Geometry check sheet. Reference: the model listing, model coordinates, mm. Face numbers are marked on the shaded views. A direction names the side the tool comes from. Give positions to 0.01 mm unless a question says otherwise; leave off trailing zeros. Write each loop counter-clockwise with the first axis right and the second up, starting at its lowest first coordinate (ties: lowest second). Pieces come first, ordered by that corner, then holes. Notation, with made-up numbers: M 28.5,51.25 L 34.5,51.25 A25 cw 34.5,66.25 Z; hole C 62,50.5 d7. An arc over 180 degrees is marked long. One line per item, written item: value. Start each with the question number.
1. Tool access check on the marked faces 4, 5 and 6. Record the directions out of +Z, -Z, +X, -X, +Y, -Y that give a thin tool (end or side, any length) a straight path to the whole face; none if there is none.
2. Cross-section at A-A on y = -9. Count the separate pieces of the cut face and the enclosed holes in it, then the cut area to 3 significant figures.
3. Cross-section at C-C on z = 7.5. Record the cut outline in (x, y).
4. Gauge pin test, flat ends, axial feed: pin 1 (4 mm diameter, centred on x = 22, y = -3.5, fed in from -Z); pin 2 (1.5 mm diameter, centred on x = -16.5, y = -9, fed in from +Z); pin 3 (1.5 mm diameter, centred on x = -6.5, y = -10, fed in from -Z). Record the tip position at first contact, or that the pin passes through.
5. Cross-section at B-B on x = 4.5. Record the cut outline in (y, z).
6. Scan lines: line 1 (X direction, y = -6.35, z = -7.3); line 2 (X direction, y = -6.35, z = -7.4); line 3 (X direction, y = -7.25, z = -8). Record each from-to range of solid material in increasing order.
7. Cross-section at D-D on z = 11.25. Record the cut outline in (x, y).
8. Release check for a two-part mould opening along X. For the marked faces 1, 2 and 3 record: pulls with the +X half, pulls with the -X half, needs draft (parallel to the pull), parting line crosses it, or undercut.
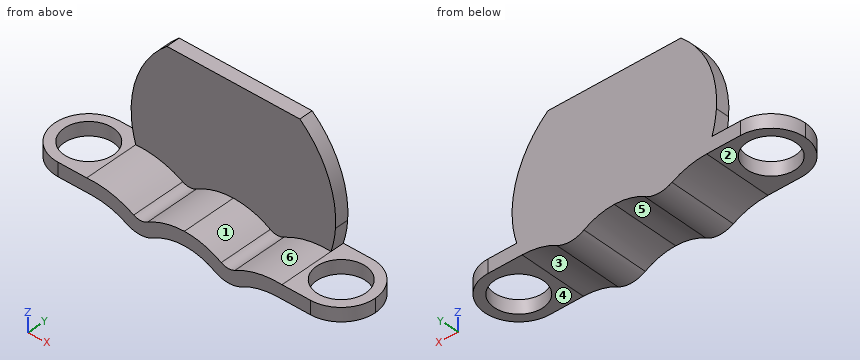
from build123d import *

# Parameters (mm, degrees)
F1_DEPTH = 2.54
F2_DEPTH = 12.7
F3_R     = 5.08
F5_DEPTH = 25.4
F7_R     = 2.54


with BuildPart() as f1:
    # F0 (on Front) → F1 (new body)
    with BuildSketch(Plane.XZ):
        with BuildLine():
            Line((12.3829699, 14.4763447201), (-12.3829699, 14.4763447201))
            ThreePointArc((-12.3829699, 14.4763447201), (-17.5494163181, 7.4108357757), (-19.0109455672, -1.2192))
            ThreePointArc((-19.0109455672, -1.2192), (-18.7320588508, -3.4659012121), (-18.1886103823, -5.6636518574))
            ThreePointArc((-18.1886103823, -5.6636518574), (-12.9594922672, -6.2044133907), (-8.1898528707, -8.414987824))
            ThreePointArc((-8.1898528707, -8.414987824), (-0.0244050051, -5.6637208939), (8.1261735346, -8.4587303814))
            ThreePointArc((8.1261735346, -8.4587303814), (12.9222610069, -6.2147067253), (18.1886103823, -5.6636518574))
            ThreePointArc((18.1886103823, -5.6636518574), (18.7320588508, -3.4659012121), (19.0109455672, -1.2192))
            ThreePointArc((19.0109455672, -1.2192), (17.5494163181, 7.4108357757), (12.3829699, 14.4763447201))
        make_face()
    extrude(amount=F1_DEPTH)

    # F0 (on Front) → F2 (join)
    with BuildSketch(Plane.XZ):
        with BuildLine():
            ThreePointArc((-8.1898528707, -8.414987824), (-12.9594922672, -6.2044133907), (-18.1886103823, -5.6636518574))
            Line((-18.1886103823, -5.6636518574), (-29.86024, -5.6636518574))
            Line((-29.86024, -5.6636518574), (-29.86024, -8.2036518574))
            Line((-29.86024, -8.2036518574), (-17.1930973418, -8.2036518574))
            ThreePointArc((-17.1930973418, -8.2036518574), (-12.3090033163, -9.1264565308), (-8.0982998954, -11.7676531566))
            ThreePointArc((-8.0982998954, -11.7676531566), (-0.0191744615, -8.2037507277), (8.0326972664, -11.8288065861))
            ThreePointArc((8.0326972664, -11.8288065861), (12.2672793977, -9.1428876591), (17.1930973418, -8.2036518574))
            Line((17.1930973418, -8.2036518574), (29.86024, -8.2036518574))
            Line((29.86024, -8.2036518574), (29.86024, -5.6636518574))
            Line((29.86024, -5.6636518574), (18.1886103823, -5.6636518574))
            ThreePointArc((18.1886103823, -5.6636518574), (12.9222610069, -6.2147067253), (8.1261735346, -8.4587303814))
            ThreePointArc((8.1261735346, -8.4587303814), (-0.0244050051, -5.6637208939), (-8.1898528707, -8.414987824))
        make_face()
    extrude(amount=F2_DEPTH)

    # F3
    f3_edges = [f1.edges().sort_by_distance(p)[0] for p in [
        (-8.0983, -6.35, -11.767653),
        (8.032697, -6.35, -11.828807),
    ]]
    fillet(f3_edges, radius=F3_R)

    # F4 (on face) → F5 (cut)
    with BuildSketch(Plane.XY.offset(-5.6636518574)):
        with BuildLine():
            ThreePointArc((-18.93824, -6.35), (-23.51024, -1.778), (-28.08224, -6.35))
            ThreePointArc((-28.08224, -6.35), (-23.51024, -10.922), (-18.93824, -6.35))
        make_face()
        with BuildLine():
            Line((-29.86024, 0), (-29.86024, -6.35))
            ThreePointArc((-29.86024, -6.35), (-28.0003680605, -1.8598719395), (-23.51024, 0))
            Line((-23.51024, 0), (-29.86024, 0))
        make_face()
        with BuildLine():
            ThreePointArc((-23.51024, -12.7), (-28.0003680605, -10.8401280605), (-29.86024, -6.35))
            Line((-29.86024, -6.35), (-29.86024, -12.7))
            Line((-29.86024, -12.7), (-23.51024, -12.7))
        make_face()
    extrude(amount=-F5_DEPTH, mode=Mode.SUBTRACT)

    # F6: F1 across plane


with BuildPart() as f1_1:
    add(f1.part)
    add(f1.part.mirror(Plane.YZ), mode=Mode.INTERSECT)

    # F7
    f7_edges = [f1_1.edges().sort_by_distance(p)[0] for p in [
        (-8.126174, -7.62, -8.45873),
        (8.126174, -7.62, -8.45873),
    ]]
    fillet(f7_edges, radius=F7_R)


solid = f1_1.part
Report:
1. face 4: -Z, +X, +Y, -Y
1. face 5: -Z, +Y, -Y
1. face 6: +Z, -Y
2. separate pieces: 3
2. enclosed holes: 0
2. area: 115 mm^2
3. outline: M -17.51,-2.54 L 17.51,-2.54 L 17.51,0 L -17.51,0 Z
4. pin 1: stops at z = -8.2
4. pin 2: stops at z = -5.63
4. pin 3: stops at z = -10.39
5. outline: M -12.7,-9.15 L 0,-9.15 L 0,14.48 L -2.54,14.48 L -2.54,-6.46 L -12.7,-6.46 Z
6. line 1: x = -29.86 to -28.08, -18.94 to -10.09, -6.35 to 6.35, 10.09 to 18.94, 28.08 to 29.86
6. line 2: x = -29.86 to -28.08, -18.94 to -9.89, -6.53 to 6.53, 9.89 to 18.94, 28.08 to 29.86
6. line 3: x = -29.8 to -27.99, -19.03 to 19.03, 27.99 to 29.8
7. outline: M -15.37,-2.54 L 15.37,-2.54 L 15.37,0 L -15.37,0 Z
8. face 1: undercut
8. face 2: needs draft
8. face 3: pulls with the +X half
